Work out the finished part from the listing and answer in its coordinate system (mm). A direction names the side the tool comes from. Round coordinates to 2 decimals unless told otherwise and drop trailing zeros. Order: outer loops, then holes, each group sorted by start corner. A loop starts at its lowest first (then second) coordinate and runs counter-clockwise, first axis right, second up.
from build123d import *

# Parameters (mm, degrees)
BOSS_EXTRUDE2_DEPTH = 7
SKETCH2_R           = 4
BOSS_EXTRUDE3_DEPTH = 7.8
SKETCH3_R           = 1.25
CUT_EXTRUDE1_DEPTH  = 7.8
FILLET1_R           = 3
FILLET2_R           = 3
CUT_EXTRUDE2_DEPTH  = 1


with BuildPart() as part:
    # Sketch1 → Boss-Extrude2 (new body)
    with BuildSketch(Plane.XY):
        Polygon((-34.5, 0), (34.5, 0), (37.5, 15), (45.5, 15), (45.5, 21), (34.5, 21), (32.581176584, 21), (29.581176584, 6), (-29.581176584, 6), (-32.581176584, 21), (-45.5, 21), (-45.5, 15), (-37.5, 15), align=None)
    extrude(amount=BOSS_EXTRUDE2_DEPTH)

    # Sketch2 → Boss-Extrude3 (add)
    with BuildSketch(Plane(origin=(0, 21, 0), x_dir=(1, 0, 0), z_dir=(0, 1, 0))):
        with Locations((45.5, -3.5)):
            Circle(SKETCH2_R)
    boss_extrude3 = extrude(amount=-BOSS_EXTRUDE3_DEPTH)

    # Mirror1: Boss-Extrude3 across plane
    add(boss_extrude3.mirror(Plane(origin=(0, 0, 0), x_dir=(0, 0, 1), z_dir=(1, 0, 0))))

    # Sketch3 → Cut-Extrude1 (cut)
    with BuildSketch(Plane(origin=(0, 21, 0), x_dir=(1, 0, 0), z_dir=(0, 1, 0))):
        with Locations((45.5, -3.5)):
            Circle(SKETCH3_R)
    cut_extrude1 = extrude(amount=-CUT_EXTRUDE1_DEPTH, mode=Mode.SUBTRACT)

    # Mirror2: Cut-Extrude1 across plane
    add(cut_extrude1.mirror(Plane(origin=(0, 0, 0), x_dir=(0, 0, 1), z_dir=(1, 0, 0))), mode=Mode.SUBTRACT)

    # Fillet1
    fillet1_edges = [part.edges().sort_by_distance(p)[0] for p in [
        (34.5, 0, 3.5),
        (29.581176584, 6, 3.5),
    ]]
    fillet(fillet1_edges, radius=FILLET1_R)

    # Fillet2
    fillet2_edges = [part.edges().sort_by_distance(p)[0] for p in [
        (37.5, 15, 3.5),
        (-34.5, 0, 3.5),
        (-37.5, 15, 3.5),
        (-32.581176584, 21, 3.5),
        (-29.581176584, 6, 3.5),
        (32.581176584, 21, 3.5),
    ]]
    fillet(fillet2_edges, radius=FILLET2_R)

    # Sketch4 → Cut-Extrude2 (cut)
    with BuildSketch(Plane.XY.offset(7)):
        with BuildLine():
            Line((-36.037089005, 12.784464541), (-34.001749643, 2.60776773))
            ThreePointArc((-34.001749643, 2.60776773), (-33.308566103, 1.453315717), (-32.040588292, 1))
            Line((-32.040588292, 1), (32.040588292, 1))
            ThreePointArc((32.040588292, 1), (33.308566103, 1.453315717), (34.001749643, 2.60776773))
            Line((34.001749643, 2.60776773), (36.037089005, 12.784464541))
            ThreePointArc((36.037089005, 12.784464541), (37.423456086, 15.093368565), (39.959411708, 16))
            Line((39.959411708, 16), (42.563508327, 16))
            Line((42.563508327, 16), (42.563508327, 20))
            Line((42.563508327, 20), (35.040588292, 20))
            ThreePointArc((35.040588292, 20), (33.772610481, 19.546684283), (33.07942694, 18.39223227))
            Line((33.07942694, 18.39223227), (31.044087578, 8.215535459))
            ThreePointArc((31.044087578, 8.215535459), (29.657720498, 5.906631435), (27.121764876, 5))
            Line((27.121764876, 5), (-27.121764876, 5))
            ThreePointArc((-27.121764876, 5), (-29.657720498, 5.906631435), (-31.044087578, 8.215535459))
            Line((-31.044087578, 8.215535459), (-33.07942694, 18.39223227))
            ThreePointArc((-33.07942694, 18.39223227), (-33.772610481, 19.546684283), (-35.040588292, 20))
            Line((-35.040588292, 20), (-42.563508327, 20))
            Line((-42.563508327, 20), (-42.563508327, 16))
            Line((-42.563508327, 16), (-39.959411708, 16))
            ThreePointArc((-39.959411708, 16), (-37.423456086, 15.093368565), (-36.037089005, 12.784464541))
        make_face()
    extrude(amount=-CUT_EXTRUDE2_DEPTH, mode=Mode.SUBTRACT)


solid = part.part
Item 1: Find section A-A (z = 3.5). State how many separate pieces and enclosed holes the cut face has, plus the area to 3 significant figures.
Item 2: Given pin 1 (3 mm diameter, centred on x = 45.5, z = 3.5, fed in from -Y); pin 2 (6.5 mm diameter, centred on x = 2.5, y = 8.5, fed in from +Z); pin 3 (3 mm diameter, centred on x = 34, z = 1, fed in from -Y), each flat-ended and moving along its own axis, determine where each tip first touches the part or whether it passes through.
Item 3: For a pull along Y with two mould halves and no side action, classify faces 1 (the face through (38.08, 14.34, 3.55)), 2 (the face through (33.79, 19.56, 6.51)), 3 (the face through (-33.116, 20.302, 3.549)), 4 (the face through (32.076, 13.375, 6.507)) as released by +Y, released by -Y, zero draft, split by the parting line, or undercut.
Item 4: Find the intervals of material crossed by line 1 along Y through (x, z) = (-26.5, 6.25); line 2 along X through (y, z) = (18.25, 3.5); line 3 along Z through (x, y) = (45.5, 19.5), in increasing order.
Item 5: A tool of negligible diameter and unlimited length cuts with its end or side. For faces 5 (the face through (-33.758, 19.534, 6.507)), 6 (the face through (41, 15, 3)), 7 (the face through (33.116, 20.302, 3.549)), from which of +Z, -Z, +X, -X, +Y, -Y can it reach the whole face along a straight path? Write none if from no direction.
Item 6: Find section C-C (y = 9.75). Write down the section's boundary in (x, z), plus the area to 3 significant figures.
Item 7: Find section D-D (x = 14). Write down the section's boundary in (y, z), plus the area to 3 significant figures.
Item 8: Find section B-B (x = 45.5). Write down the section's boundary in (y, z), plus the area to 3 significant figures.
Model answer:
1. separate pieces: 3
1. enclosed holes: 0
1. area: 731 mm2
2. pin 1: stops at y = 13.2
2. pin 2: stops at z = 7
2. pin 3: stops at y = 0.04
3. face 1: released by -Y
3. face 2: undercut
3. face 3: released by +Y
3. face 4: undercut
4. line 1: y = 0 to 1, 5 to 6
4. line 2: x = -49.5 to -46.75, -44.25 to -32.03, 32.03 to 44.25, 46.75 to 49.5
4. line 3: z = -0.5 to 2.25, 4.75 to 7.5
5. face 5: +Z
5. face 6: -Y
5. face 7: +Z, -Z, +Y
6. outline: (-36.45, 0) - (-30.33, 0) - (-30.33, 7) - (-31.35, 7) - (-31.35, 6) - (-35.43, 6) - (-35.43, 7) - (-36.45, 7) - close; (30.33, 0) - (36.45, 0) - (36.45, 7) - (35.43, 7) - (35.43, 6) - (31.35, 6) - (31.35, 7) - (30.33, 7) - close
6. area: 77.5 mm2
7. outline: (0, 0) - (6, 0) - (6, 7) - (5, 7) - (5, 6) - (1, 6) - (1, 7) - (0, 7) - close
7. area: 38.0 mm2
8. outline: (13.2, -0.5) - (21, -0.5) - (21, 2.25) - (13.2, 2.25) - close; (13.2, 4.75) - (21, 4.75) - (21, 7.5) - (13.2, 7.5) - close
8. area: 42.9 mm2
